Autodesk Fusion 360 part; units mm, degrees
sketch "Sketch1" plane through (0, 0, -6.0198) normal (0, 0, 1) x (-1, 0, 0)
  line L0 (-4.0409, -44.45) -> (3.9347, -44.45)
  line L1 (3.9347, -44.45) -> (3.9347, 6.35)
  line L2 (3.9347, 6.35) -> (-16.6393, 6.35)
  line L3 (-16.6393, 6.35) -> (-16.6393, -44.45)
  line L4 (-16.6393, -44.45) -> (-8.6637, -44.45)
  line L5 (-8.6637, -44.45) -> (-8.6637, -42.6466)
  arc A0 (-8.1557, -42.1386) -> (-8.6637, -42.6466) centre (-8.1557, -42.6466) ccw
  line L6 (-8.1557, -42.1386) -> (-4.5489, -42.1386)
  arc A1 (-4.0409, -42.6466) -> (-4.5489, -42.1386) centre (-4.5489, -42.6466) ccw
  line L7 (-4.0409, -42.6466) -> (-4.0409, -44.45)
  arc A2 (-8.1557, -29.4386) -> (-8.6637, -29.9466) centre (-8.1557, -29.9466) ccw
  line L8 (-8.1557, -29.4386) -> (-4.5489, -29.4386)
  arc A3 (-4.0409, -29.9466) -> (-4.5489, -29.4386) centre (-4.5489, -29.9466) ccw
  line L9 (-4.0409, -29.9466) -> (-4.0409, -33.5534)
  arc A4 (-4.5489, -34.0614) -> (-4.0409, -33.5534) centre (-4.5489, -33.5534) ccw
  line L10 (-4.5489, -34.0614) -> (-8.1557, -34.0614)
  arc A5 (-8.6637, -33.5534) -> (-8.1557, -34.0614) centre (-8.1557, -33.5534) ccw
  line L11 (-8.6637, -33.5534) -> (-8.6637, -29.9466)
  arc A6 (1.8011, -40.4114) -> (2.3091, -39.9034) centre (1.8011, -39.9034) ccw
  line L12 (1.8011, -40.4114) -> (-1.8057, -40.4114)
  arc A7 (-2.3137, -39.9034) -> (-1.8057, -40.4114) centre (-1.8057, -39.9034) ccw
  line L13 (-2.3137, -39.9034) -> (-2.3137, -36.2966)
  arc A8 (-1.8057, -35.7886) -> (-2.3137, -36.2966) centre (-1.8057, -36.2966) ccw
  line L14 (-1.8057, -35.7886) -> (1.8011, -35.7886)
  arc A9 (2.3091, -36.2966) -> (1.8011, -35.7886) centre (1.8011, -36.2966) ccw
  line L15 (2.3091, -36.2966) -> (2.3091, -39.9034)
  arc A10 (1.8011, -27.7114) -> (2.3091, -27.2034) centre (1.8011, -27.2034) ccw
  line L16 (1.8011, -27.7114) -> (-1.8057, -27.7114)
  arc A11 (-2.3137, -27.2034) -> (-1.8057, -27.7114) centre (-1.8057, -27.2034) ccw
  line L17 (-2.3137, -27.2034) -> (-2.3137, -23.5966)
  arc A12 (-1.8057, -23.0886) -> (-2.3137, -23.5966) centre (-1.8057, -23.5966) ccw
  line L18 (-1.8057, -23.0886) -> (1.8011, -23.0886)
  arc A13 (2.3091, -23.5966) -> (1.8011, -23.0886) centre (1.8011, -23.5966) ccw
  line L19 (2.3091, -23.5966) -> (2.3091, -27.2034)
  arc A14 (1.8011, -15.0114) -> (2.3091, -14.5034) centre (1.8011, -14.5034) ccw
  line L20 (1.8011, -15.0114) -> (-1.8057, -15.0114)
  arc A15 (-2.3137, -14.5034) -> (-1.8057, -15.0114) centre (-1.8057, -14.5034) ccw
  line L21 (-2.3137, -14.5034) -> (-2.3137, -10.8966)
  arc A16 (-1.8057, -10.3886) -> (-2.3137, -10.8966) centre (-1.8057, -10.8966) ccw
  line L22 (-1.8057, -10.3886) -> (1.8011, -10.3886)
  arc A17 (2.3091, -10.8966) -> (1.8011, -10.3886) centre (1.8011, -10.8966) ccw
  line L23 (2.3091, -10.8966) -> (2.3091, -14.5034)
  arc A18 (1.8011, -2.3114) -> (2.3091, -1.8034) centre (1.8011, -1.8034) ccw
  line L24 (1.8011, -2.3114) -> (-1.8057, -2.3114)
  arc A19 (-2.3137, -1.8034) -> (-1.8057, -2.3114) centre (-1.8057, -1.8034) ccw
  line L25 (-2.3137, -1.8034) -> (-2.3137, 1.8034)
  arc A20 (-1.8057, 2.3114) -> (-2.3137, 1.8034) centre (-1.8057, 1.8034) ccw
  line L26 (-1.8057, 2.3114) -> (1.8011, 2.3114)
  arc A21 (2.3091, 1.8034) -> (1.8011, 2.3114) centre (1.8011, 1.8034) ccw
  line L27 (2.3091, 1.8034) -> (2.3091, -1.8034)
  arc A22 (-10.8989, -40.4114) -> (-10.3909, -39.9034) centre (-10.8989, -39.9034) ccw
  line L28 (-10.8989, -40.4114) -> (-14.5057, -40.4114)
  arc A23 (-15.0137, -39.9034) -> (-14.5057, -40.4114) centre (-14.5057, -39.9034) ccw
  line L29 (-15.0137, -39.9034) -> (-15.0137, -36.2966)
  arc A24 (-14.5057, -35.7886) -> (-15.0137, -36.2966) centre (-14.5057, -36.2966) ccw
  line L30 (-14.5057, -35.7886) -> (-10.8989, -35.7886)
  arc A25 (-10.3909, -36.2966) -> (-10.8989, -35.7886) centre (-10.8989, -36.2966) ccw
  line L31 (-10.3909, -36.2966) -> (-10.3909, -39.9034)
  arc A26 (-10.8989, -27.7114) -> (-10.3909, -27.2034) centre (-10.8989, -27.2034) ccw
  line L32 (-10.8989, -27.7114) -> (-14.5057, -27.7114)
  arc A27 (-15.0137, -27.2034) -> (-14.5057, -27.7114) centre (-14.5057, -27.2034) ccw
  line L33 (-15.0137, -27.2034) -> (-15.0137, -23.5966)
  arc A28 (-14.5057, -23.0886) -> (-15.0137, -23.5966) centre (-14.5057, -23.5966) ccw
  line L34 (-14.5057, -23.0886) -> (-10.8989, -23.0886)
  arc A29 (-10.3909, -23.5966) -> (-10.8989, -23.0886) centre (-10.8989, -23.5966) ccw
  line L35 (-10.3909, -23.5966) -> (-10.3909, -27.2034)
  arc A30 (-10.8989, -15.0114) -> (-10.3909, -14.5034) centre (-10.8989, -14.5034) ccw
  line L36 (-10.8989, -15.0114) -> (-14.5057, -15.0114)
  arc A31 (-15.0137, -14.5034) -> (-14.5057, -15.0114) centre (-14.5057, -14.5034) ccw
  line L37 (-15.0137, -14.5034) -> (-15.0137, -10.8966)
  arc A32 (-14.5057, -10.3886) -> (-15.0137, -10.8966) centre (-14.5057, -10.8966) ccw
  line L38 (-14.5057, -10.3886) -> (-10.8989, -10.3886)
  arc A33 (-10.3909, -10.8966) -> (-10.8989, -10.3886) centre (-10.8989, -10.8966) ccw
  line L39 (-10.3909, -10.8966) -> (-10.3909, -14.5034)
  arc A34 (-10.8989, -2.3114) -> (-10.3909, -1.8034) centre (-10.8989, -1.8034) ccw
  line L40 (-10.8989, -2.3114) -> (-14.5057, -2.3114)
  arc A35 (-15.0137, -1.8034) -> (-14.5057, -2.3114) centre (-14.5057, -1.8034) ccw
  line L41 (-15.0137, -1.8034) -> (-15.0137, 1.8034)
  arc A36 (-14.5057, 2.3114) -> (-15.0137, 1.8034) centre (-14.5057, 1.8034) ccw
  line L42 (-14.5057, 2.3114) -> (-10.8989, 2.3114)
  arc A37 (-10.3909, 1.8034) -> (-10.8989, 2.3114) centre (-10.8989, 1.8034) ccw
  line L43 (-10.3909, 1.8034) -> (-10.3909, -1.8034)
  arc A38 (-8.6637, -8.1534) -> (-8.1557, -8.6614) centre (-8.1557, -8.1534) ccw
  line L44 (-8.6637, -8.1534) -> (-8.6637, -4.5466)
  arc A39 (-8.1557, -4.0386) -> (-8.6637, -4.5466) centre (-8.1557, -4.5466) ccw
  line L45 (-8.1557, -4.0386) -> (-4.5489, -4.0386)
  arc A40 (-4.0409, -4.5466) -> (-4.5489, -4.0386) centre (-4.5489, -4.5466) ccw
  line L46 (-4.0409, -4.5466) -> (-4.0409, -8.1534)
  arc A41 (-4.5489, -8.6614) -> (-4.0409, -8.1534) centre (-4.5489, -8.1534) ccw
  line L47 (-4.5489, -8.6614) -> (-8.1557, -8.6614)
  arc A42 (-8.1557, -16.7386) -> (-8.6637, -17.2466) centre (-8.1557, -17.2466) ccw
  line L48 (-8.1557, -16.7386) -> (-4.5489, -16.7386)
  arc A43 (-4.0409, -17.2466) -> (-4.5489, -16.7386) centre (-4.5489, -17.2466) ccw
  line L49 (-4.0409, -17.2466) -> (-4.0409, -20.8534)
  arc A44 (-4.5489, -21.3614) -> (-4.0409, -20.8534) centre (-4.5489, -20.8534) ccw
  line L50 (-4.5489, -21.3614) -> (-8.1557, -21.3614)
  arc A45 (-8.6637, -20.8534) -> (-8.1557, -21.3614) centre (-8.1557, -20.8534) ccw
  line L51 (-8.6637, -20.8534) -> (-8.6637, -17.2466)
  line L52 (1.3947, -23.5966) -> (-14.0993, -23.5966)
  line L53 (-16.6393, -21.0566) -> (-16.6393, 19.5834)
  line L54 (-14.0993, 22.1234) -> (1.3947, 22.1234)
  line L55 (3.9347, 19.5834) -> (3.9347, -21.0566)
  arc A46 (1.3947, -23.5966) -> (3.9347, -21.0566) centre (1.3947, -21.0566) ccw
  arc A47 (-16.6393, -21.0566) -> (-14.0993, -23.5966) centre (-14.0993, -21.0566) ccw
  arc A48 (-14.0993, 22.1234) -> (-16.6393, 19.5834) centre (-14.0993, 19.5834) ccw
  arc A49 (3.9347, 19.5834) -> (1.3947, 22.1234) centre (1.3947, 19.5834) ccw
  circle A50 centre (-6.3523, 14.0389) radius 4.191
  point P0 (3.9347, -23.5966)
  point P1 (-16.6393, -23.5966)
  point P2 (3.9347, 22.1234)
  dimension "d1" = 20.574
  dimension "d2" = 45.72
  dimension "d3" = 2.54
  dimension "d4" = 8.382
extrude "Extrude1" add sketch "Sketch1" along normal blind 6.35 contours L1 L2 L3 A12 L18 A13 A28 L34 A29 L52 L53 L55 A46 A47 | L2 L53 L54 L55 A48 A49 | A12 L18 A13 L52 A46 | A28 L34 A29 L52 A47
Check sheet for the modelled part. Datum: model origin and axes. Units: mm. A direction names the side the tool comes from. Give positions to 0.01 mm unless a question says otherwise; leave off trailing zeros. Loops run counter-clockwise (first coordinate to the right, second up) from the corner with the lowest first, then second, coordinate; pieces in that order, holes last. Notation, with made-up numbers: M -6.5,28 L 34.5,28 A19 cw 34.5,43 Z; hole C -12.5,85.25 d8. An arc over 180 degrees is marked long. Answer as CSV lines item,"result".
Item 1: Sectioned sample at A-A, the plane x = 13. Enter the section's corners in (y, z).
Reply:
outline,"M -22.12,-6.02 L -2.31,-6.02 L -2.31,0.33 L -22.12,0.33 Z; M 2.31,-6.02 L 10.39,-6.02 L 10.39,0.33 L 2.31,0.33 Z; M 15.01,-6.02 L 23.6,-6.02 L 23.6,0.33 L 15.01,0.33 Z"
Item 2: Scan lines: L1, parallel to Y at x = 12.5, z = -5; L2, parallel to X at y = 0, z = -0.5; L3, parallel to Y at x = 4.25, z = -2.5. Record each from-to range of solid material in increasing order.
Reply:
L1,"-22.12 to -2.31, 2.31 to 10.39, 15.01 to 23.6"
L2,"-3.93 to -2.31, 2.31 to 10.39, 15.01 to 16.64"
L3,"-22.12 to -17.66, -10.41 to 4.14, 8.56 to 16.84, 21.26 to 23.6"
Item 3: Depth check by flat-ended pin: pin 1 Ø5 at (x, y) = (6.35, -14.04) entering from +Z. Enter the tip coordinate at first touch or a pass-through.
Reply:
pin 1,"through"
Item 4: Set-up check for faces 5 (the face through (16.639, 0, -3)), 6 (the face through (15.014, 13, -3)): record each of +Z, -Z, +X, -X, +Y, -Y from which the full face is reachable in a straight line by a thin tool's end or side.
Reply:
face 5,"+Z, -Z, +X, +Y, -Y"
face 6,"+Z, -Z"
Item 5: Sectioned sample at B-B, the plane y = 0. Enter the section's corners in (x, z), then the cut area to 3 significant figures.
Reply:
outline,"M -3.93,-6.02 L -2.31,-6.02 L -2.31,0.33 L -3.93,0.33 Z; M 2.31,-6.02 L 10.39,-6.02 L 10.39,0.33 L 2.31,0.33 Z; M 15.01,-6.02 L 16.64,-6.02 L 16.64,0.33 L 15.01,0.33 Z"
area,"71.9 mm^2"
Item 6: Draft check along Y on faces 1 (the face through (6, 0, -6.02)), 2 (the face through (2.314, 13, -3)), 3 (the face through (-3.21, 22.833, -2.889)), 4 (the face through (0, 2.311, -3)). Enter one of: pulls with the +Y half, pulls with the -Y half, needs draft (parallel to the pull), parting line crosses it, or undercut.
Reply:
face 1,"needs draft"
face 2,"undercut"
face 3,"pulls with the +Y half"
face 4,"undercut"
Item 7: Sectioned sample at D-D, the plane x = 5.5. Enter the section's corners in (y, z).
Reply:
outline,"M -22.12,-6.02 L -18.14,-6.02 L -18.14,0.33 L -22.12,0.33 Z; M -9.94,-6.02 L 4.04,-6.02 L 4.04,0.33 L -9.94,0.33 Z; M 8.66,-6.02 L 16.74,-6.02 L 16.74,0.33 L 8.66,0.33 Z; M 21.36,-6.02 L 23.6,-6.02 L 23.6,0.33 L 21.36,0.33 Z"
Item 8: Sectioned sample at C-C, the plane y = 20. Enter the section's corners in (x, z), then the cut area to 3 significant figures.
Reply:
outline,"M -3.93,-6.02 L 4.04,-6.02 L 4.04,0.33 L -3.93,0.33 Z; M 8.66,-6.02 L 16.64,-6.02 L 16.64,0.33 L 8.66,0.33 Z"
area,"101 mm^2"
